Part model, mm, in its own coordinate system. Give positions to 0.01 mm unless a question says otherwise; leave off trailing zeros. Write each loop counter-clockwise with the first axis right and the second up, starting at its lowest first coordinate (ties: lowest second). Pieces come first, ordered by that corner, then holes. Notation, with made-up numbers: M -38.5,2 L 6.5,2 A29 ccw 6.5,35 Z; hole C 36,-24 d5. An arc over 180 degrees is marked long. Use CSV: the item, a comma, the result in double quotes. Start each with the question number.
1. Drill centre lines: line 1 along X through (y, z) = (1.35, 0); line 2 along X through (y, z) = (4.35, 0); line 3 along Z through (x, y) = (10, 5.4). Where is each one in solid material? Low to high. Write a range as from..to.
2. Band-saw the part on B-B, the plane y = 5. List the corners of the cut face in (x, z), then the cut area to 3 significant figures.
3. Drop flat-ended pins along their axis: pin 1 Ø8.5 at (x, z) = (155, 0) entering from +Y; pin 2 Ø4 at (x, z) = (6.5, 3.5) entering from +Y. Give the stop position or say it passes through.
4. Band-saw the part on C-C, the plane z = 0. Count the separate pieces of the cut face and the enclosed holes in it, then the cut area to 3 significant figures.
5. Band-saw the part on A-A, the plane x = 10. List the corners of the cut face in (y, z).
from build123d import *

# Parameters (mm, degrees)
SKETCH1_W           = 165
SKETCH1_H           = 20
BOSS_EXTRUDE1_DEPTH = 10
CHAMFER1_SIZE       = 5


with BuildPart() as part:
    # Sketch1 → Boss-Extrude1 (new body)
    with BuildSketch(Plane(origin=(0, 0, 0), x_dir=(1, 0, 0), z_dir=(0, 1, 0))):
        with Locations((82.5, 0)):
            Rectangle(SKETCH1_W, SKETCH1_H)
    extrude(amount=BOSS_EXTRUDE1_DEPTH)

    # Chamfer1
    chamfer1_edges = [part.edges().sort_by_distance(p)[0] for p in [
        (0, 5, -10),
        (165, 5, -10),
        (165, 5, 10),
        (0, 5, 10),
    ]]
    chamfer(chamfer1_edges, length=CHAMFER1_SIZE)

    # Sketch2 → Cut-Revolve1 (revolve, cut)
    with BuildSketch(Plane.XY):
        Polygon((2.7, 7), (3, 7), (3, 2), (5, 2), (5, 0), (10, 0), (10, 10), (3, 10), (3, 8.15), (2.7, 8.15), align=None)
    revolve(axis=Axis((10, 10, 0), (0, -1, 0)), mode=Mode.SUBTRACT)

    # Sketch7 → Cut-Revolve2 (revolve, cut)
    with BuildSketch(Plane.XY, mode=Mode.PRIVATE) as cut_revolve2_sk:
        Polygon((148, 10), (148, 8.15), (147.7, 8.15), (147.7, 7), (148, 7), (148, 2), (150, 2), (150, 0), (155, 0), (155, 10), align=None)
    revolve(cut_revolve2_sk.sketch.rotate(Axis((155, 10, 0), (0, -1, 0)), 270), axis=Axis((155, 10, 0), (0, -1, 0)), mode=Mode.SUBTRACT)


solid = part.part
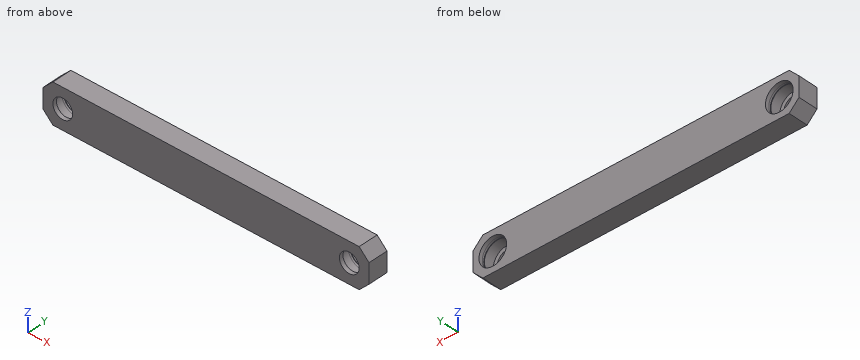
Output:
1,line 1,"x = 0..5, 15..150, 160..165"
1,line 2,"x = 0..3, 17..148, 162..165"
1,line 3,"z = -10..-7, 7..10"
2,outline,"M 0,-5 L 5,-10 L 160,-10 L 165,-5 L 165,5 L 160,10 L 5,10 L 0,5 Z; hole C 10,0 d14; hole C 155,0 d14"
2,area,"2,940 mm²"
3,pin 1,"passes through"
3,pin 2,"stops at y = 2"
4,separate pieces,"3"
4,enclosed holes,"0"
4,area,"1,380 mm²"
5,outline,"M 0,-10 L 10,-10 L 10,-7 L 8.15,-7 L 8.15,-7.3 L 7,-7.3 L 7,-7 L 2,-7 L 2,-5 L 0,-5 Z; M 0,5 L 2,5 L 2,7 L 7,7 L 7,7.3 L 8.15,7.3 L 8.15,7 L 10,7 L 10,10 L 0,10 Z"
